```python
from build123d import *

# Parameters (mm, degrees)
EXTRUDE_1_DEPTH          = 300
CUT_EXTRUDE_1_DEPTH      = 1.0000001
CUT_EXTRUDE_1_DEPTH_BACK = 831.0000001
SKETCH_4_W               = 15
SKETCH_4_H               = 45
CUT_EXTRUDE_2_DEPTH      = 243.720162759
SKETCH_4_3_W             = 15
SKETCH_4_3_H             = 45
CUT_EXTRUDE_3_DEPTH      = 10


with BuildPart() as part:
    # 스케치1 → 보스-돌출1 (new body)
    with BuildSketch(Plane(origin=(0, 0, 0), x_dir=(0, 0, -1), z_dir=(1, 0, 0))):
        with BuildLine():
            Line((-41.993007726, 32.892860384), (-41.993007726, -303.619075042))
            Line((-41.993007726, -303.619075042), (788.006992274, -303.619075042))
            Line((788.006992274, -303.619075042), (788.006992274, -12.90547458))
            add(Edge.make_bspline(
                [(788.006992274, -12.90547458), (680.261509472, 78.254339674), (631.210016853, 128.415858034), (368.750142796, 135.255878696)],
                knots=[0, 0, 0, 0, 1, 1, 1, 1], degree=3))
            add(Edge.make_bspline(
                [(45.325655749, 132.198658827), (134.989620851, 137.211386353), (265.463569923, 138.011524869), (368.750142796, 135.255878696)],
                knots=[0, 0, 0, 0, 1, 1, 1, 1], degree=3))
            Line((45.325655749, 132.198658827), (-41.993007726, 32.892860384))
        make_face()
        with BuildLine():
            Line((4.116595834, 54.214584045), (54.427658026, 114.389853292))
            add(Edge.make_bspline(
                [(54.427658026, 114.389853292), (122.914694658, 118.068796405), (254.727094278, 116.434615788), (344.321994749, 115.599177573)],
                knots=[0, 0, 0, 0, 0.843637698, 0.843637698, 0.843637698, 0.843637698], degree=3))
            Line((344.321994749, 115.599177573), (359.116595834, -53.619075042))
            Line((359.116595834, -53.619075042), (4.116595834, -53.619075042))
            Line((4.116595834, -53.619075042), (4.116595834, 54.214584045))
        make_face(mode=Mode.SUBTRACT)
        with BuildLine():
            Line((414.932922958, -53.619075042), (389.116595834, 115.255878696))
            add(Edge.make_bspline(
                [(389.116595834, 115.255878696), (584.597474826, 110.825479528), (668.447748965, 84.913988672), (744.116595834, 1.380924958)],
                knots=[0.027735734, 0.027735734, 0.027735734, 0.027735734, 0.842070206, 0.842070206, 0.842070206, 0.842070206], degree=3))
            Line((744.116595834, 1.380924958), (744.116595834, -53.619075042))
            Line((744.116595834, -53.619075042), (414.932922958, -53.619075042))
        make_face(mode=Mode.SUBTRACT)
    extrude(amount=EXTRUDE_1_DEPTH)

    # 스케치2 → 컷-돌출1 (cut, two sides)
    with BuildSketch(Plane.XY.offset(41.993007726)) as cut_extrude_1_sk:
        Polygon((179.652203691, 32.892860384), (239.655287588, 136.821250303), (265.636049701, 121.821250303), (214.293219842, 32.892860384), (300, 32.892860384), (300, -303.619075042), (341.364714008, -303.619075042), (341.364714008, 251.457374482), (0, 251.457374482), (0, 32.892860384), align=None)
        Polygon((95.31772029, -113.178749697), (179.652203691, 32.892860384), (0, 32.892860384), (0, -303.619075042), (95.31772029, -303.619075042), align=None)
        Polygon((300, 32.892860384), (214.293219842, 32.892860384), (129.958736441, -113.178749697), (129.958736441, -303.619075042), (300, -303.619075042), align=None)
    extrude(amount=CUT_EXTRUDE_1_DEPTH, mode=Mode.SUBTRACT)
    extrude(cut_extrude_1_sk.sketch, amount=-CUT_EXTRUDE_1_DEPTH_BACK, mode=Mode.SUBTRACT)

    # 스케치4 → 컷-돌출2 (cut, through all)
    with BuildSketch(Plane(origin=(120.496126421, -69.568471025, 0), x_dir=(0, 0, 1), z_dir=(-0.866025404, 0.5, 0))):
        with Locations((-374.116595834, 175.489898801)):
            Rectangle(SKETCH_4_W, SKETCH_4_H)
    extrude(amount=-CUT_EXTRUDE_2_DEPTH, mode=Mode.SUBTRACT)

    # 스케치4<3> → 컷-돌출3 (cut)
    with BuildSketch(Plane(origin=(120.496126421, -69.568471025, 0), x_dir=(0, 0, 1), z_dir=(-0.866025404, 0.5, 0))):
        Polygon((-744.116595834, 18.416776129), (-744.116595834, 213.416776129), (-389.116595834, 213.416776129), (-389.116595834, 17.989898801), (-389.116595834, -11.583223871), (-744.116595834, -11.583223871), align=None)
        Polygon((-359.116595834, 18.416776129), (-359.116595834, 212.989898801), (-4.116595834, 212.989898801), (-4.116595834, 17.989898801), (-4.116595834, -12.010101199), (-359.116595834, -12.010101199), align=None)
        with Locations((-374.116595834, 175.489898801)):
            Rectangle(SKETCH_4_3_W, SKETCH_4_3_H)
    extrude(amount=-CUT_EXTRUDE_3_DEPTH, mode=Mode.SUBTRACT)


solid = part.part
```
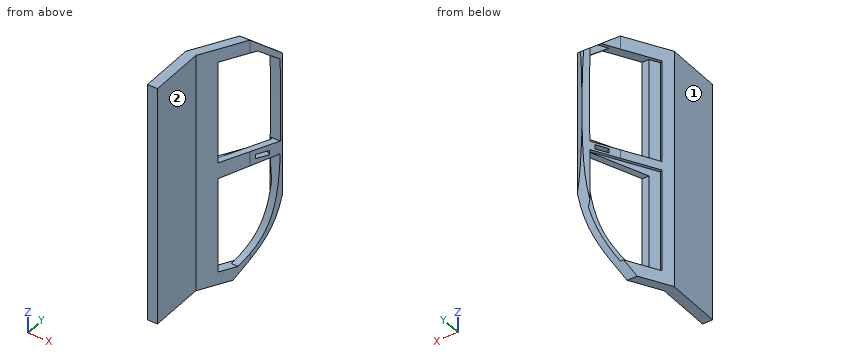
Check sheet for the modelled part. Datum: model origin and axes. Units: mm. Face numbers are marked on the shaded views. A direction names the side the tool comes from. Give positions to 0.01 mm unless a question says otherwise; leave off trailing zeros. Write each loop counter-clockwise with the first axis right and the second up, starting at its lowest first coordinate (ties: lowest second). Pieces come first, ordered by that corner, then holes. Notation, with made-up numbers: (-7.5, 23.25) - (8.5, 23.25) arc R17 cw to (8.5, 32.25) - close; hole circle Ø8 at (73, -39.75). An arc over 180 degrees is marked (long way). Answer as a JSON object with one key per item and string values. Group by question number.
1) Sectioned sample at B-B (y = -100). Record the cut outline in (x, z).
2) Thickness scan on probe 1 along X at (y, z) = (-80.5, -667); probe 2 along X at (y, z) = (-249.5, -650); probe 3 along Y at (x, z) = (229.5, -518.5). Record the ranges inside material, lowest first. Write a range as from..to.
3) Access from +Z, -Z, +X, -X, +Y, -Y to the whole of each face (thin tool, end or side, straight path). Record for the marked faces 1 and 2.
4) Depth check by flat-ended pin: P1, Ø11.5, axis at x = 149.5, z = -534, coming from the +Y side; P2, Ø1.5, axis at x = 136.5, z = -173, coming from the -Y side; P3, Ø6, axis at y = -125, z = -586, coming from the +X side. Enter the tip coordinate at first touch or a pass-through.
5) Sectioned sample at A-A (y = 77). Give the number of separate pieces and of enclosed holes in the cut face, then the cut area to 3 significant figures.
Geometry results:
{
 "1": {"outline": "(102.93, -788.01) - (137.57, -788.01) - (137.57, 41.99) - (102.93, 41.99) - close"},
 "2": {"probe 1": "x = 114.18..116.26, 125.73..148.83", "probe 2": "x = 95.32..129.96", "probe 3": "y = 113.93..119.23"},
 "3": {"face 1": "+Z, -Z, -X, +Y, -Y", "face 2": "+Z, -Z, +X, -Y"},
 "4": {"P1": "stops at y = -53.62", "P2": "stops at y = -103.15", "P3": "stops at x = 129.96"},
 "5": {"separate pieces": "4", "enclosed holes": "0", "area": "2,250 mm^2"}
}
